Geometry check sheet. Reference: the model listing, model coordinates, mm. Face numbers are marked on the shaded views. A direction names the side the tool comes from. Give positions to 0.01 mm unless a question says otherwise; leave off trailing zeros. Order: outer loops, then holes, each group sorted by start corner. A loop starts at its lowest first (then second) coordinate and runs counter-clockwise, first axis right, second up. Notation, with made-up numbers: M 19.5,34 L 72.5,34 A6 ccw 72.5,38 Z; hole C 70.25,26 d7. An arc over 180 degrees is marked long. Answer as CSV lines item,"result". Start each with the question number.
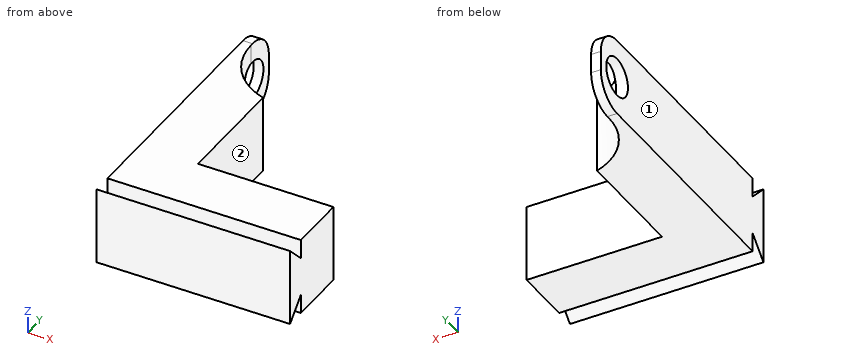
```python
from build123d import *

# Parameters (mm, degrees)
SKETCH1_W           = 8
SKETCH1_H           = 30
BOSS_EXTRUDE1_DEPTH = 6
SKETCH2_W           = 8
SKETCH2_H           = 10
CUT_EXTRUDE1_DEPTH  = 5
CUT_EXTRUDE2_REACH  = 18.643
SKETCH3_R           = 2
FILLET1_R           = 3
FILLET2_R           = 7
SKETCH4_W           = 8
SKETCH4_H           = 8
BOSS_EXTRUDE2_DEPTH = 14
CUT_EXTRUDE4_REACH  = 27.318


with BuildPart() as part:
    # Sketch1 → Boss-Extrude1 (new body)
    with BuildSketch(Plane(origin=(0, 0, 0), x_dir=(0, 0, -1), z_dir=(1, 0, 0))):
        Rectangle(SKETCH1_W, SKETCH1_H)
    extrude(amount=BOSS_EXTRUDE1_DEPTH)

    # Sketch2 → Cut-Extrude1 (cut)
    with BuildSketch(Plane(origin=(6, 0, 0), x_dir=(0, 0, -1), z_dir=(1, 0, 0))):
        with Locations((0, 10)):
            Rectangle(SKETCH2_W, SKETCH2_H)
    extrude(amount=-CUT_EXTRUDE1_DEPTH, mode=Mode.SUBTRACT)

    # Sketch3 → Cut-Extrude2 (cut, up to next)
    with BuildSketch(Plane.ZY, mode=Mode.PRIVATE) as cut_extrude2_sk1:
        with Locations((0, 12)):
            Circle(SKETCH3_R)
    cut_extrude2_tool1 = extrude(cut_extrude2_sk1.sketch, amount=-CUT_EXTRUDE2_REACH, mode=Mode.PRIVATE) & part.part
    add(cut_extrude2_tool1.solids().sort_by_distance((0, 12, 0))[0], mode=Mode.SUBTRACT)

    # Fillet1
    fillet1_edges = [part.edges().sort_by_distance(p)[0] for p in [
        (0.5, 15, 4),
        (0.5, 15, -4),
    ]]
    fillet(fillet1_edges, radius=FILLET1_R)

    # Fillet2
    # the kernel refuses this fillet: 7 mm, written as the material it adds along each edge
    with BuildSketch(Plane(origin=(1, 5, 4), x_dir=(0, 1, 0), z_dir=(0, 0, -1))) as fillet2_piece_1_section:
        with BuildLine():
            CenterArc((6.708203932, 7), FILLET2_R, 196.601549599, 73.398450401)
            Line((0, 5), (0, 0))
            Line((0, 0), (6.708203932, 0))
        make_face()
    fillet2_piece_1 = extrude(amount=8, mode=Mode.PRIVATE)
    fillet2_piece_1 = fillet2_piece_1 - Plane(origin=(1, 12, 0), x_dir=(0, 0, 1), z_dir=(-1, 0, 0)) * Cylinder(2, 43, mode=Mode.PRIVATE)
    add(fillet2_piece_1)

    # Sketch4 → Boss-Extrude2 (add)
    with BuildSketch(Plane(origin=(6, 0, 0), x_dir=(0, 0, -1), z_dir=(1, 0, 0))):
        with Locations((0, -11)):
            Rectangle(SKETCH4_W, SKETCH4_H)
    extrude(amount=BOSS_EXTRUDE2_DEPTH)

    # Sketch6 → Cut-Extrude4 (cut, up to next)
    with BuildSketch(Plane.ZY, mode=Mode.PRIVATE) as cut_extrude4_sk1:
        Polygon((4, -15), (4, -13), (2, -13), align=None)
    cut_extrude4_tool1 = extrude(cut_extrude4_sk1.sketch, amount=-CUT_EXTRUDE4_REACH, mode=Mode.PRIVATE) & part.part
    # Sketch6 → Cut-Extrude4 (cut, up to next)
    with BuildSketch(Plane.ZY, mode=Mode.PRIVATE) as cut_extrude4_sk2:
        Polygon((-4, -15), (-4, -13), (-2, -13), align=None)
    cut_extrude4_tool2 = extrude(cut_extrude4_sk2.sketch, amount=-CUT_EXTRUDE4_REACH, mode=Mode.PRIVATE) & part.part
    add(cut_extrude4_tool1.solids().sort_by_distance((0, -13.666667, 3.333333))[0], mode=Mode.SUBTRACT)
    add(cut_extrude4_tool2.solids().sort_by_distance((0, -13.666667, -3.333333))[0], mode=Mode.SUBTRACT)


solid = part.part
```
Item 1: Section check D-D on y = 9.5. Record the boundary of the cut face in (x, z), then the cut area to 3 significant figures.
Item 2: Section check A-A on z = 0. Record the boundary of the cut face in (x, y), then the cut area to 3 significant figures.
Item 3: Section check B-B on x = 9. Record the boundary of the cut face in (y, z), then the cut area to 3 significant figures.
Item 4: Depth check by flat-ended pin: pin 1 Ø1 at (y, z) = (3.5, -1) entering from +X; pin 2 Ø2.5 at (x, z) = (14.5, -1) entering from +Y; pin 3 Ø2.5 at (y, z) = (13.5, -0.5) entering from +X. Enter the tip coordinate at first touch or a pass-through.
Item 5: Access from +Z, -Z, +X, -X, +Y, -Y to the whole of each face (thin tool, end or side, straight path). Record for the marked faces 1 and 2.
Item 6: Scan lines: line 1 along Y through (x, z) = (0.35, 0); line 2 along Z through (x, y) = (0.7, 12); line 3 along Y through (x, z) = (18.75, 0). Record each from-to range of solid material in increasing order.
Item 7: Section check C-C on z = -3.5. Record the boundary of the cut face in (x, y), then the cut area to 3 significant figures.
Numbers:
1,outline,"M 0,-4 L 1.36,-4 L 1.36,4 L 0,4 Z"
1,area,"10.9 mm2"
2,outline,"M 0,-15 L 20,-15 L 20,-7 L 6,-7 L 6,5 A7 cw 1.21,10 L 0,10 Z; M 0,14 L 1,14 L 1,15 L 0,15 Z"
2,area,"247 mm2"
3,outline,"M -15,-4 L -13,-2 L -13,-4 L -7,-4 L -7,4 L -13,4 L -13,2 L -15,4 Z"
3,area,"60.0 mm2"
4,pin 1,"x = 6"
4,pin 2,"y = -7"
4,pin 3,"x = 1"
5,face 1,"+Z, -Z, -X, +Y, -Y"
5,face 2,"+Z, -Z, +X, +Y"
6,line 1,"-15 to 10, 14 to 15"
6,line 2,"-4 to -2, 2 to 4"
6,line 3,"-15 to -7"
7,outline,"M 0,-15 L 20,-15 L 20,-14.5 L 0,-14.5 Z; M 0,-13 L 20,-13 L 20,-7 L 6,-7 L 6,5 A7 cw 1,11.71 L 1,13.66 L 0,13.66 Z"
7,area,"220 mm2"
